Input: part model. Units: mm. Frame: model coordinates. A direction names the side the tool comes from. Round coordinates to 2 decimals unless told otherwise and drop trailing zeros. Write each loop counter-clockwise with the first axis right and the second up, starting at its lowest first coordinate (ties: lowest second). Pieces come first, ordered by that corner, then holes. Notation, with made-up numbers: (31, -27.5) -> (54, -27.5) arc R15 ccw to (54, -16.5) -> close; hole circle Ø1 at (17.5, 54.5). An arc over 180 degrees is marked (long way). Use CSV: the item, a comma, the result in double quotes.
```python
from build123d import *

# Parameters (mm, degrees)
F0_R     = 2
F1_DEPTH = 5


with BuildPart() as f1:
    # F0 (on Top) → F1 (new body)
    with BuildSketch(Plane.XY):
        with BuildLine():
            ThreePointArc((-3.8750014305, 0), (-4.2267672199, -2.1093164988), (-5.2439909973, -3.9903298027))
            Line((-5.2439909973, -3.9903298027), (5.6694109986, -12.4775612749))
            ThreePointArc((5.6694109986, -12.4775612749), (9.8825038634, -12.9132287637), (12.1249985695, -9.3200163929))
            Line((12.1249985695, -9.3200163929), (12.1249985695, 9.3200163929))
            ThreePointArc((12.1249985695, 9.3200163929), (9.8825038634, 12.9132287637), (5.6694109986, 12.4775612749))
            Line((5.6694109986, 12.4775612749), (-5.2439909973, 3.9903298027))
            ThreePointArc((-5.2439909973, 3.9903298027), (-4.2267672199, 2.1093164988), (-3.8750014305, 0))
        make_face()
        Polygon((8.0675292322, 2.2068999953), (6.0064843484, -3.8768709144), (5.756569483, -3.8768709144), (4.1200787681, 0.4710455388), (2.4399282273, -3.8768709144), (2.1900133619, -3.8768709144), (0.1018692759, 2.2068999953), (-0.449147837, 2.3288464056), (-0.449147837, 2.5787612709), (1.9596701426, 2.5787612709), (1.9596701426, 2.3288464056), (1.0337807317, 2.2068999953), (2.5347754353, -2.2388746883), (4.2329921109, 2.1361409672), (4.4437636841, 2.1361409672), (6.0817599103, -2.2388746883), (7.5119955856, 2.2068999953), (6.5288967477, 2.3288464056), (6.5288967477, 2.5787612709), (8.6170408338, 2.5787612709), (8.6170408338, 2.3288464056), align=None, mode=Mode.SUBTRACT)
        with BuildLine():
            ThreePointArc((-15.5059721811, 3.9903808286), (-16.8750014304, 3.23201e-05), (-15.5060118637, -3.9903298027))
            ThreePointArc((-15.5060118637, -3.9903298027), (-10.3750014305, -6.5), (-5.2439909973, -3.9903298027))
            ThreePointArc((-5.2439909973, -3.9903298027), (-4.2267672199, -2.1093164988), (-3.8750014305, 0))
            ThreePointArc((-3.8750014305, 0), (-4.2267672199, 2.1093164988), (-5.2439909973, 3.9903298027))
            ThreePointArc((-5.2439909973, 3.9903298027), (-10.3749691104, 6.4999999999), (-15.5059721811, 3.9903808286))
        make_face()
        with BuildLine():
            Line((-10.3772096263, -2.9674286779), (-10.9801440776, -2.9674286779))
            Line((-10.9801440776, -2.9674286779), (-10.9801440776, -4.7481291549))
            Line((-10.9801440776, -4.7481291549), (-10.1293933476, -4.8554310488))
            Line((-10.1293933476, -4.8554310488), (-10.1293933476, -5.0674800295))
            Line((-10.1293933476, -5.0674800295), (-12.385287926, -5.0674800295))
            Line((-12.385287926, -5.0674800295), (-12.385287926, -4.8554310488))
            Line((-12.385287926, -4.8554310488), (-11.7504183872, -4.7481291549))
            Line((-11.7504183872, -4.7481291549), (-11.7504183872, -0.0294006313))
            Line((-11.7504183872, -0.0294006313), (-12.4376614694, 0.0740690521))
            Line((-12.4376614694, 0.0740690521), (-12.4376614694, 0.2861180328))
            Line((-12.4376614694, 0.2861180328), (-10.4168091348, 0.2861180328))
            add(Edge.make_bspline(
                [(-10.4168091348, 0.2861180328), (-8.4534399575, 0.2861180328), (-8.4534399575, -1.2914752879)],
                knots=[0, 0, 0, 1, 1, 1], degree=2))
            add(Edge.make_bspline(
                [(-8.4534399575, -1.2914752879), (-8.4534399575, -2.1128457374), (-8.9503499185, -2.5401372077)],
                knots=[0, 0, 0, 1, 1, 1], degree=2))
            add(Edge.make_bspline(
                [(-8.9503499185, -2.5401372077), (-9.4472598794, -2.9674286779), (-10.3772096263, -2.9674286779)],
                knots=[0, 0, 0, 1, 1, 1], degree=2))
        make_face(mode=Mode.SUBTRACT)
        with Locations((-10.3750014305, 3.25)):
            Circle(F0_R, mode=Mode.SUBTRACT)
        with BuildLine():
            Line((-32.8750014305, 9.3202724501), (-32.8750014305, -9.3200163929))
            ThreePointArc((-32.8750014305, -9.3200163929), (-30.6325067245, -12.9132287637), (-26.4194138596, -12.4775612749))
            Line((-26.4194138596, -12.4775612749), (-15.5060118637, -3.9903298027))
            ThreePointArc((-15.5060118637, -3.9903298027), (-16.8750014304, 3.23201e-05), (-15.5059721811, 3.9903808286))
            Line((-15.5059721811, 3.9903808286), (-26.4193824591, 12.477792912))
            ThreePointArc((-26.4193824591, 12.477792912), (-30.6324888578, 12.9134935598), (-32.8750014305, 9.3202724501))
        make_face()
        with BuildLine():
            Line((-28.1915230864, -4.0461723693), (-28.1915230864, -3.7470318405))
            Line((-28.1915230864, -3.7470318405), (-27.2220194448, -3.5956595247))
            Line((-27.2220194448, -3.5956595247), (-27.2220194448, 3.0611182673))
            Line((-27.2220194448, 3.0611182673), (-28.1915230864, 3.2070844289))
            Line((-28.1915230864, 3.2070844289), (-28.1915230864, 3.5062249578))
            Line((-28.1915230864, 3.5062249578), (-22.5258735526, 3.5062249578))
            Line((-22.5258735526, 3.5062249578), (-22.5258735526, 1.6987674252))
            Line((-22.5258735526, 1.6987674252), (-22.8970961366, 1.6987674252))
            Line((-22.8970961366, 1.6987674252), (-23.0773012744, 2.9205582598))
            add(Edge.make_bspline(
                [(-23.0773012744, 2.9205582598), (-23.7080192569, 2.9980464691), (-24.9027793208, 2.9980464691)],
                knots=[0, 0, 0, 1, 1, 1], degree=2))
            Line((-24.9027793208, 2.9980464691), (-26.1353824636, 2.9980464691))
            Line((-26.1353824636, 2.9980464691), (-26.1353824636, 0.0480883625))
            Line((-26.1353824636, 0.0480883625), (-24.0972623546, 0.0480883625))
            Line((-24.0972623546, 0.0480883625), (-23.9224633709, 0.9491140518))
            Line((-23.9224633709, 0.9491140518), (-23.5620530952, 0.9491140518))
            Line((-23.5620530952, 0.9491140518), (-23.5620530952, -1.3719281237))
            Line((-23.5620530952, -1.3719281237), (-23.9224633709, -1.3719281237))
            Line((-23.9224633709, -1.3719281237), (-24.0972623546, -0.4582880748))
            Line((-24.0972623546, -0.4582880748), (-26.1353824636, -0.4582880748))
            Line((-26.1353824636, -0.4582880748), (-26.1353824636, -3.5397959319))
            Line((-26.1353824636, -3.5397959319), (-24.6486900764, -3.5397959319))
            add(Edge.make_bspline(
                [(-24.6486900764, -3.5397959319), (-23.1962366654, -3.5397959319), (-22.7457238208, -3.449693363)],
                knots=[0, 0, 0, 1, 1, 1], degree=2))
            Line((-22.7457238208, -3.449693363), (-22.4249586754, -2.0531035447))
            Line((-22.4249586754, -2.0531035447), (-22.0519340401, -2.0531035447))
            Line((-22.0519340401, -2.0531035447), (-22.1600571228, -4.0461723693))
            Line((-22.1600571228, -4.0461723693), (-28.1915230864, -4.0461723693))
        make_face(mode=Mode.SUBTRACT)
    extrude(amount=F1_DEPTH)


solid = f1.part
```
Item 1: Section query A-A on y = 4.5. Return the cut outline in (x, z) (3 decimals), plus the area to 3 significant figures.
Worked answers:
outline,"(-32.875, 0) -> (-16.161, 0) -> (-16.161, 5) -> (-32.875, 5) -> close; (-15.065, 0) -> (-11.936, 0) -> (-11.936, 5) -> (-15.065, 5) -> close; (-8.814, 0) -> (-5.685, 0) -> (-5.685, 5) -> (-8.814, 5) -> close; (-4.589, 0) -> (12.125, 0) -> (12.125, 5) -> (-4.589, 5) -> close"
area,"198 mm²"
Item 2: Section query C-C on x = 5. Return the cut outline in (y, z).
Worked answers:
outline,"(-11.96, 0) -> (-1.87, 0) -> (-1.87, 5) -> (-11.96, 5) -> close; (0.65, 0) -> (11.96, 0) -> (11.96, 5) -> (0.65, 5) -> close"
Item 3: Set-up query: faces 1 (the face through (3.292, -1.672, 2.465)), 2 (the face through (-20.886, 8.175, 2.465)), 3 (the face through (-10.5, -6.5, 2.5)). Return all of +Z, -Z, +X, -X, +Y, -Y with unobstructed straight access to the full face (end or side cutting, diameter ignored); none if empty.
Worked answers:
face 1,"+Z, -Z"
face 2,"+Z, -Z, +Y"
face 3,"+Z, -Z, -Y"
Item 4: Section query B-B on y = -10. Return the cut outline in (x, z), plus the area to 3 significant figures.
Worked answers:
outline,"(-32.82, 0) -> (-23.23, 0) -> (-23.23, 5) -> (-32.82, 5) -> close; (2.48, 0) -> (12.07, 0) -> (12.07, 5) -> (2.48, 5) -> close"
area,"95.8 mm²"
Item 5: Line query: line 1 (X direction, y = -2.5, z = 4.1) (3 decimals); line 2 (Y direction, x = -9, z = 2.95); line 3 (X direction, y = -3, z = 2.7) (3 decimals). Output: solid intervals per line, ascending.
Worked answers:
line 1,"x = -32.875 to -27.222, -26.135 to -22.528, -22.076 to -11.75, -8.906 to 1.717, 2.972 to 5.238, 6.473 to 12.125"
line 2,"y = -6.35 to -2.58, -0.07 to 1.8, 4.7 to 6.35"
line 3,"x = -32.875 to -27.222, -26.135 to -22.642, -22.103 to -11.75, -10.98 to 1.889, 2.779 to 5.427, 6.304 to 12.125"
Item 6: Pull-direction query (Y, two-part tool) for faces 4 (the face through (0.136, -8.175, 2.465)), 5 (the face through (6.8, 0, 2.5)), 6 (the face through (-10.3, 6.5, 2.5)); classes: +Y half, -Y half, draft (parallel to the pull), parting line (faces both ways), or undercut.
Worked answers:
face 4,"-Y half"
face 5,"undercut"
face 6,"+Y half"
Item 7: Section query D-D on z = 0.8. Give the number of separate pieces and of enclosed holes in the cut face, plus the area to 3 significant figures.
Worked answers:
separate pieces,"1"
enclosed holes,"4"
area,"748 mm²"
Item 8: First-contact query: pin 1 Ø4.5 at (x, y) = (-10.38, 3.25) entering from +Z; pin 2 Ø1.2 at (x, z) = (-25.5, 2) entering from -Y; pin 3 Ø1.6 at (x, z) = (-12, 1.5) entering from -Y. Flat tips, straight axial feed; report the tip coordinate or a pass-through.
Worked answers:
pin 1,"stops at z = 5"
pin 2,"stops at y = -12.23"
pin 3,"stops at y = -6.45"
